Could you check a few things on this model? Use its own coordinates, in mm. A direction names the side the tool comes from. Round coordinates to 2 decimals unless told otherwise and drop trailing zeros. Write each loop counter-clockwise with the first axis right and the second up, starting at its lowest first coordinate (ties: lowest second). Pieces come first, ordered by that corner, then holes. Notation, with made-up numbers: (-28, 75.5) -> (-11, 75.5) arc R23 ccw to (-11, 98.5) -> close; hole circle Ø1 at (20.25, 85.25). An arc over 180 degrees is marked (long way). Answer as CSV lines item,"result". Start each with the question number.
Q1. Imagine slicing it at C-C on z = -21.5. Give the number of separate pieces and of enclosed holes in the cut face, and give its area (3 significant figures).
Q2. Imagine slicing it at B-B on z = 10. Please give me the cut outline in (x, y) (3 decimals), and give its area (3 significant figures).
Q3. If we mould it in two halves opening along Z, with no side actions, what happens to faces 3 (the flat face through (30, 2, 10)), 4 (the cylindrical face through (0, 3, 13)), 5 (the flat face through (20, 2, -20))? For each: pulls with the +Z half, pulls with the -Z half, needs draft (parallel to the pull), parting line crosses it, or undercut.
Q4. For faces 1 (the flat face through (-20, 2, -20)), 2 (the conical face through (8, 2.6, -17)), which set-ups out of +Z, -Z, +X, -X, +Y, -Y let a thin tool reach every point of the face, with its end or its side?
Q5. If I drill on line 1 (X direction, y = 2.7, z = 10); line 2 (Z direction, x = 0, y = 2.65), over which ranges is the centre line in solid material (lowest first)? Write a range as [from, to].
Q6. Will these pins go through, and if not, where does the flat tip stop? pin 1 Ø1.5 at (x, y) = (18.5, 3) entering from -Z; pin 2 Ø4.5 at (x, z) = (10, -10) entering from +Y; pin 3 Ø2 at (x, y) = (-18.5, 4) entering from -Z.
Q7. Imagine slicing it at A-A on x = 0. Please give me the cut outline in (y, z) (3 decimals), and give its area (3 significant figures).
from build123d import *

# Parameters (mm, degrees)
EXTRUDE_1_DEPTH                = 5
HOLE_WIZARD_M3_1_2_D           = 3.4
HOLE_WIZARD_M3_1_2_CSINK_D     = 3.45
HOLE_WIZARD_M3_1_2_CSINK_ANGLE = 90


with BuildPart() as part:
    # 草图1 → 凸台-拉伸1 (new body)
    with BuildSketch(Plane(origin=(0, 0, 0), x_dir=(1, 0, 0), z_dir=(0, 1, 0))):
        Polygon((-10, 30), (-30, 10), (-30, -30), (30, -30), (30, 10), (10, 30), align=None)
    extrude(amount=EXTRUDE_1_DEPTH)

    # 草图8 → Hole Wizard M3 _1 (revolve, cut)
    with BuildSketch(Plane(origin=(-15.656854249, 2.5, -24.343145751), x_dir=(-0.707106781186551, 0, 0.707106781186544), z_dir=(0, 1, 0))):
        Polygon((0, 0), (0, 10.751075774), (1.25, 10), (1.25, 0.025), (1.275, 0), align=None)
    hole_wizard_m3_1 = revolve(axis=Axis((-20.14698231, 2.5, -28.833273811), (0.707106781186544, 0, 0.707106781186551)), mode=Mode.SUBTRACT)

    # 草图10 → M16 螺纹孔的螺纹孔钻头1 (revolve, cut)
    with BuildSketch(Plane(origin=(0, 5, 20), x_dir=(0, 0, 1), z_dir=(1, 0, 0))):
        Polygon((0, 0), (0, 5), (7, 5), (7, 0.025), (7.025, 0), align=None)
    revolve(axis=Axis((0, 11.35, 20), (0, -1, 0)), mode=Mode.SUBTRACT)

    # 镜向2: Hole Wizard M3 _1 across plane
    add(hole_wizard_m3_1.mirror(Plane(origin=(0, 0, 0), x_dir=(0, 0, 1), z_dir=(1, 0, 0))), mode=Mode.SUBTRACT)

    # Hole Wizard M3 _1 2 (through all)
    with Locations(Plane(origin=(-10, 5, -10), x_dir=(0, 0, 1), z_dir=(0, 1, 0))):
        with Locations((0, 0), (0, 20), (20, 20), (20, 0)):
            CounterSinkHole(HOLE_WIZARD_M3_1_2_D / 2, HOLE_WIZARD_M3_1_2_CSINK_D / 2, counter_sink_angle=HOLE_WIZARD_M3_1_2_CSINK_ANGLE)


solid = part.part
Checks:
1,separate pieces,"1"
1,enclosed holes,"2"
1,area,"171 mm^2"
2,outline,"(-30, 0) -> (-11.7, 0) -> (-11.7, 4.975) -> (-11.725, 5) -> (-30, 5) -> close; (-8.3, 0) -> (8.3, 0) -> (8.3, 4.975) -> (8.275, 5) -> (-8.275, 5) -> (-8.3, 4.975) -> close; (11.7, 0) -> (30, 0) -> (30, 5) -> (11.725, 5) -> (11.7, 4.975) -> close"
2,area,"266 mm^2"
3,face 3,"needs draft"
3,face 4,"undercut"
3,face 5,"pulls with the -Z half"
4,face 1,"-Z, -X, +Y, -Y"
4,face 2,"none"
5,line 1,"[-30, -11.7], [-8.3, 8.3], [11.7, 30]"
5,line 2,"[-30, 13], [27, 30]"
6,pin 1,"z = -22.25"
6,pin 2,"y = 5"
6,pin 3,"z = -22.5"
7,outline,"(0, -30) -> (5, -30) -> (5, 12.975) -> (4.975, 13) -> (0, 13) -> close; (0, 27) -> (4.975, 27) -> (5, 27.025) -> (5, 30) -> (0, 30) -> close"
7,area,"230 mm^2"
